Can you work these out from the model? Positions are in its coordinate system, mm. Face numbers are marked on the shaded views. A direction names the side the tool comes from. Give positions to 0.01 mm unless a question says otherwise; leave off trailing zeros. Order: outer loops, then holes, each group sorted by start corner. A loop starts at its lowest first (then second) coordinate and runs counter-clockwise, first axis right, second up. Notation, with made-up numbers: M 33,-20.75 L 70,-20.75 A22 cw 70,-9.75 Z; hole C 55,65 d8. An arc over 180 degrees is marked long. Write each question's results on one line, items separated by ' | '.
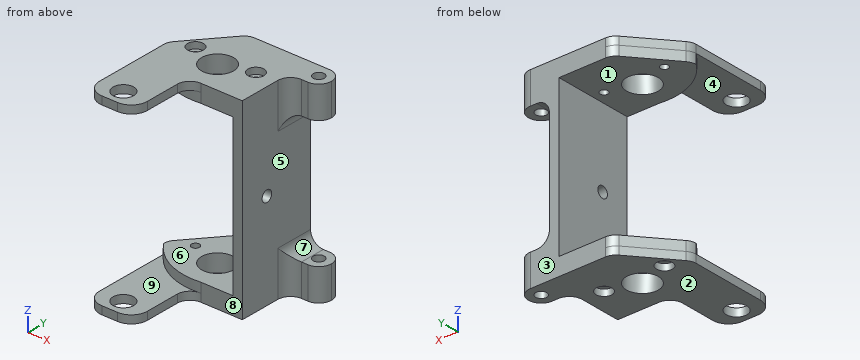
from build123d import *

# Parameters (mm, degrees)
BOSS_EXTRUDE1_DEPTH      = 30
BOSS_EXTRUDE1_DEPTH_BACK = 30
SKETCH2_R                = 3.25
SKETCH2_R_2              = 1.25
SKETCH2_R_3              = 5
SKETCH3_W                = 58
SKETCH3_H                = 55
CUT_EXTRUDE1_DEPTH       = 60.373815778
SKETCH4_W                = 10
SKETCH4_H                = 8
BOSS_EXTRUDE2_DEPTH      = 10
FILLET1_R                = 4
SKETCH5_R                = 1.75
CUT_EXTRUDE2_DEPTH       = 76.599272483
FILLET1_OF_MIRROR1_R     = 4
FILLET2_R                = 4
SKETCH6_R                = 1.25
SKETCH6_R_2              = 5
BOSS_EXTRUDE3_DEPTH      = 3
SKETCH7_R                = 2.5
CUT_EXTRUDE3_DEPTH       = 2
SKETCH8_R                = 1.75
CUT_EXTRUDE4_DEPTH       = 63.841069373


with BuildPart() as part:
    # Sketch2 → Boss-Extrude1 (new, two sides: drawn at the far end of the back side and taken through both)
    with BuildSketch(Plane.XY.offset(-BOSS_EXTRUDE1_DEPTH_BACK)):
        with BuildLine():
            Line((-7.5, 5), (-7.5, 30))
            Line((-7.5, 30), (5.086494468, 45))
            Line((5.086494468, 45), (24.5, 45))
            Line((24.5, 45), (24.5, 20))
            Line((24.5, 20), (7.5, 20))
            Line((7.5, 20), (7.5, 5))
            ThreePointArc((7.5, 5), (6.035533906, 1.464466094), (2.5, 0))
            Line((2.5, 0), (-2.5, 0))
            ThreePointArc((-2.5, 0), (-6.035533906, 1.464466094), (-7.5, 5))
        make_face()
        with Locations((0, 5)):
            Circle(SKETCH2_R, mode=Mode.SUBTRACT)
        with Locations((18.004770913, 32.569673822)):
            Circle(SKETCH2_R_2, mode=Mode.SUBTRACT)
        with Locations((-0.995229087, 32.569673822)):
            Circle(SKETCH2_R_2, mode=Mode.SUBTRACT)
        with Locations((8.504770913, 29.569673822)):
            Circle(SKETCH2_R_3, mode=Mode.SUBTRACT)
    extrude(amount=BOSS_EXTRUDE1_DEPTH + BOSS_EXTRUDE1_DEPTH_BACK)

    # Sketch3 → Cut-Extrude1 (cut, through all)
    with BuildSketch(Plane(origin=(0, 45, 0), x_dir=(1, 0, 0), z_dir=(0, 1, 0))):
        with Locations((-7.5, 0)):
            Rectangle(SKETCH3_W, SKETCH3_H)
    extrude(amount=-CUT_EXTRUDE1_DEPTH, mode=Mode.SUBTRACT)

    # Sketch4 → Boss-Extrude2 (add)
    with BuildSketch(Plane(origin=(24.5, 0, 0), x_dir=(0, 0, -1), z_dir=(1, 0, 0))):
        with Locations((-25, 41)):
            Rectangle(SKETCH4_W, SKETCH4_H)
    boss_extrude2 = extrude(amount=BOSS_EXTRUDE2_DEPTH)

    # Fillet1
    fillet1_edges = [part.edges().sort_by_distance(p)[0] for p in [
        (34.5, 37, 25),
        (34.5, 45, 25),
    ]]
    fillet(fillet1_edges, radius=FILLET1_R - 0.0001)  # a hair under: the kernel refuses the full size

    # Sketch5 → Cut-Extrude2 (cut, through all)
    with BuildSketch(Plane(origin=(0, 0, 20), x_dir=(-1, 0, 0), z_dir=(0, 0, -1))):
        with Locations((-30.5, 41)):
            Circle(SKETCH5_R)
    cut_extrude2 = extrude(amount=-CUT_EXTRUDE2_DEPTH, mode=Mode.SUBTRACT)

    # Mirror1: Boss-Extrude2, Cut-Extrude2 across plane
    add(boss_extrude2.mirror(Plane.XY))
    add(cut_extrude2.mirror(Plane.XY), mode=Mode.SUBTRACT)

    # Fillet1 of Mirror1
    fillet1_of_mirror1_edges = [part.edges().sort_by_distance(p)[0] for p in [
        (34.5, 37, -25),
        (34.5, 45, -25),
    ]]
    fillet(fillet1_of_mirror1_edges, radius=FILLET1_OF_MIRROR1_R - 0.0001)  # a hair under: the kernel refuses the full size

    # Fillet2
    fillet2_edges = [part.edges().sort_by_distance(p)[0] for p in [
        (24.5, 37, 25),
        (24.5, 41, 20),
        (24.5, 37, -25),
        (24.5, 41, -20),
        (5.086494468, 45, -28.75),
        (7.5, 20, -28.75),
        (-7.5, 30, -28.75),
        (-7.5, 30, 28.75),
        (7.5, 20, 28.75),
        (5.086494468, 45, 28.75),
    ]]
    fillet(fillet2_edges, radius=FILLET2_R)

    # Sketch6 → Boss-Extrude3 (add)
    with BuildSketch(Plane.XY.offset(-27.5)):
        with BuildLine():
            Line((21.5, 45), (6.9517251, 45))
            ThreePointArc((6.9517251, 45), (5.261252053, 44.625231148), (3.887547328, 43.571150439))
            Line((3.887547328, 43.571150439), (-6.564177772, 31.115269502))
            ThreePointArc((-6.564177772, 31.115269502), (-7.258770483, 29.912199636), (-7.5, 28.544119063))
            ThreePointArc((-7.5, 28.544119063), (0.776489044, 21.551274863), (11.5, 20))
            Line((11.5, 20), (21.5, 20))
            Line((21.5, 20), (21.5, 45))
        make_face()
        with Locations((18.004770913, 32.569673822)):
            Circle(SKETCH6_R, mode=Mode.SUBTRACT)
        with Locations((8.504770913, 29.569673822)):
            Circle(SKETCH6_R_2, mode=Mode.SUBTRACT)
        with Locations((-0.995229087, 32.569673822)):
            Circle(SKETCH6_R, mode=Mode.SUBTRACT)
    boss_extrude3 = extrude(amount=BOSS_EXTRUDE3_DEPTH)

    # Sketch7 → Cut-Extrude3 (cut)
    with BuildSketch(Plane(origin=(0, 0, -30), x_dir=(-1, 0, 0), z_dir=(0, 0, -1))):
        with Locations((-18.004770913, 32.569673822)):
            Circle(SKETCH7_R)
        with Locations((0.995229087, 32.569673822)):
            Circle(SKETCH7_R)
    cut_extrude3 = extrude(amount=-CUT_EXTRUDE3_DEPTH, mode=Mode.SUBTRACT)

    # Mirror2: Boss-Extrude3, Cut-Extrude3 across plane
    add(boss_extrude3.mirror(Plane.XY))
    add(cut_extrude3.mirror(Plane.XY), mode=Mode.SUBTRACT)

    # Sketch8 → Cut-Extrude4 (cut, through all)
    with BuildSketch(Plane(origin=(24.5, 0, 0), x_dir=(0, 0, -1), z_dir=(1, 0, 0))):
        with Locations(Location((0, 29, 0), (0, 0, 90))):
            Circle(SKETCH8_R)
    extrude(amount=-CUT_EXTRUDE4_DEPTH, mode=Mode.SUBTRACT)


solid = part.part
(1) Will these pins go through, and if not, where does the flat tip stop? P1, Ø1.2, axis at y = 8.5, z = -28.5, coming from the +X side; P2, Ø3, axis at x = 9.5, y = 15.5, coming from the -Z side; P3, Ø20, axis at y = 33.5, z = -9.5, coming from the -X side; P4, Ø3, axis at x = -1, y = 32.57, coming from the -Z side.
Data:
P1: stops at x = 7.5 | P2: passes through | P3: stops at x = 21.5 | P4: stops at z = -28
(2) Imagine slicing it at D-D, the plane x = 9. Write out the boundary of the cut face in (y, z).
Data:
outline: M 19.12,-30 L 24.59,-30 L 24.59,-24.5 L 19.82,-24.5 L 19.82,-27.5 L 19.12,-27.5 Z; M 19.12,27.5 L 19.82,27.5 L 19.82,24.5 L 24.59,24.5 L 24.59,30 L 19.12,30 Z; M 34.55,-30 L 45,-30 L 45,-24.5 L 34.55,-24.5 Z; M 34.55,24.5 L 45,24.5 L 45,30 L 34.55,30 Z
(3) Imagine slicing it at B-B, the plane y = 10.5. Write out the boundary of the cut face in (x, z).
Data:
outline: M -7.5,-30 L 7.5,-30 L 7.5,-27.5 L -7.5,-27.5 Z; M -7.5,27.5 L 7.5,27.5 L 7.5,30 L -7.5,30 Z
(4) We'd pull the mould along Z, two halves only. Please class the marked faces 1, 2, 3 and 4: +Z half, -Z half, draft (parallel to the pull), parting line (faces both ways), or undercut.
Data:
face 1: undercut | face 2: -Z half | face 3: draft | face 4: undercut
(5) I need wall thicknesses on L1, parallel to Z at x = 3.5, y = 22.5; L2, parallel to Z at x = 19, y = 31; L3, parallel to X at y = 32, z = -25. Which ranges of each line are inside material? Lowest first, please. Write a range as from..to.
Data:
L1: z = -30..-24.5, 24.5..30 | L2: z = -28..-24.5, 24.5..28 | L3: x = -5.82..-2.11, 0.12..4.14, 12.87..16.89, 19.12..24.5
(6) For the marked faces 5, 6, 7, 8 and 9, which set-ups out of +Z, -Z, +X, -X, +Y, -Y let a thin tool reach every point of the face, with its end or its side?
Data:
face 5: +X, -Y | face 6: -X, +Y, -Y | face 7: +X, +Y, -Y | face 8: +Z, -Z, +X, -Y | face 9: -X, -Y
(7) Imagine slicing it at A-A, the plane z = 0. Write out the boundary of the cut face in (x, y), plus the area to 3 significant figures.
Data:
outline: M 21.5,20 L 24.5,20 L 24.5,27.25 L 21.5,27.25 Z; M 21.5,30.75 L 24.5,30.75 L 24.5,45 L 21.5,45 Z | area: 64.5 mm2
